The model under review builds one solid part; all positions refer to its coordinate system, in mm. Face numbers are marked on the shaded views. A direction names the side the tool comes from. Coordinates: 2 decimals unless noted, no trailing zeros. Order: outer loops, then holes, each group sorted by start corner. A loop starts at its lowest first (then second) coordinate and runs counter-clockwise, first axis right, second up. Notation, with made-up numbers: (-26, -15) -> (-17, -15) arc R12 ccw to (-17, 0) -> close; hole circle Ø7 at (51, -39.5). An arc over 180 degrees is marked (long way). Use one line per item in the form item = value. Start each with the question number.
(1) Insertion check: pin 1 Ø10 at (x, z) = (14.5, -59) entering from -Y; pin 2 Ø2 at (x, y) = (-59.5, 17.5) entering from +Z (3 decimals); pin 3 Ø1.5 at (y, z) = (20.5, -4) entering from -X; pin 4 Ø0.5 at (x, y) = (59.5, 17.5) entering from -Z (3 decimals). Each pin has a flat end and moves straight along its axis. Give the tip position at first contact, or say it passes through.
(2) Take a section at D-D (z = 63). State the section outline as (x, y) points.
(3) Wall thickness on line 1 along X through (y, z) = (12.5, -47.5) (3 decimals); line 2 along X through (y, z) = (17, -27) (3 decimals); line 3 along Y through (x, z) = (47, 28): over which ranges is each line inside the solid? List them lowest first.
(4) Mouldability with a two-part tool opening along Z and no side actions: class the marked faces 4, 5 and 6 as +Z half, -Z half, draft (parallel to the pull), parting line (faces both ways), or undercut.
(5) Take a section at B-B (x = 7.5). State the section outline as (y, z) points (3 decimals), then the cut area to 3 significant figures.
(6) Take a section at A-A (z = 24). State the section outline as (x, y) points (3 decimals).
(7) Take a section at C-C (x = 47). State the section outline as (y, z) points (3 decimals), then the cut area to 3 significant figures.
(8) For the marked faces 1, 2 and 3, list the 3-axis set-ups (+Z, -Z, +X, -X, +Y, -Y) from which the entire face can be reached by the end or side of a thin tool; tool diameter is ignored.
```python
from build123d import *

# Parameters (mm, degrees)
BOSS_EXTRUDE1_DEPTH     = 6.35
SKETCH3_W               = 120.65
SKETCH3_H               = 120.65
SKETCH3_W_2             = 107.95
SKETCH3_H_2             = 114.3
BOSS_EXTRUDE2_DEPTH     = 19.558
FILLET2_R               = 3.81
CUT_EXTRUDE2_DEPTH      = 52.07
CUT_EXTRUDE2_DEPTH_BACK = 39.37
FILLET3_R               = 3.81
CHAMFER1_SIZE           = 2.54


with BuildPart() as part:
    # Sketch2 → Boss-Extrude1 (new body)
    with BuildSketch(Plane(origin=(0, 0, 0), x_dir=(1, 0, 0), z_dir=(0, 1, 0))):
        with BuildLine():
            ThreePointArc((-76.2, 34.925), (-73.750256121, 26.470795103), (-66.04, 22.225))
            ThreePointArc((-66.04, 22.225), (-71.103893825, 18.75335434), (-73.66, 13.171090867))
            Line((-73.66, 13.171090867), (-73.66, -53.975))
            ThreePointArc((-73.66, -53.975), (-68.080384182, -67.445384182), (-54.61, -73.025))
            Line((-54.61, -73.025), (54.61, -73.025))
            ThreePointArc((54.61, -73.025), (68.080384182, -67.445384182), (73.66, -53.975))
            Line((73.66, -53.975), (73.66, 9.525))
            ThreePointArc((73.66, 9.525), (72.166535166, 17.2649211), (66.04, 22.225))
            ThreePointArc((66.04, 22.225), (73.750256121, 26.470795103), (76.2, 34.925))
            add(Edge.make_bspline(
                [(54.26154132, 73.334062346), (78.033661383, 68.772092229), (76.2, 34.925)],
                knots=[0, 0, 0, 1, 1, 1], degree=2))
            ThreePointArc((54.26154132, 73.334062346), (0, 79.119757765), (-54.26154132, 73.334062346))
            add(Edge.make_bspline(
                [(-54.26154132, 73.334062346), (-78.033661383, 68.772092229), (-76.2, 34.925)],
                knots=[0, 0, 0, 1, 1, 1], degree=2))
        make_face()
    extrude(amount=BOSS_EXTRUDE1_DEPTH)

    # Sketch3 → Boss-Extrude2 (add)
    with BuildSketch(Plane(origin=(0, 6.35, 0), x_dir=(1, 0, 0), z_dir=(0, 1, 0))):
        Rectangle(SKETCH3_W, SKETCH3_H)
        Rectangle(SKETCH3_W_2, SKETCH3_H_2, mode=Mode.SUBTRACT)
    extrude(amount=BOSS_EXTRUDE2_DEPTH)

    # Fillet2
    fillet2_edges = [part.edges().sort_by_distance(p)[0] for p in [
        (53.975, 6.35, 0),
        (0, 6.35, -57.15),
        (-53.975, 6.35, 0),
        (0, 6.35, 57.15),
    ]]
    fillet(fillet2_edges, radius=FILLET2_R)

    # Sketch5 → Cut-Extrude2 (cut, two sides: drawn at the far end of the back side and taken through both)
    with BuildSketch(Plane.XY.offset(-CUT_EXTRUDE2_DEPTH_BACK)):
        with BuildLine():
            Line((60.325, 21.4247353), (60.325, 12.6112647))
            ThreePointArc((60.325, 12.6112647), (58.547, 17.018), (60.325, 21.4247353))
        make_face()
        with BuildLine():
            Line((-60.325, 21.4247353), (-60.325, 12.6112647))
            ThreePointArc((-60.325, 12.6112647), (-58.547, 17.018), (-60.325, 21.4247353))
        make_face()
    extrude(amount=CUT_EXTRUDE2_DEPTH + CUT_EXTRUDE2_DEPTH_BACK, mode=Mode.SUBTRACT)

    # Fillet3
    # the kernel refuses this fillet: 3.81 mm, written as the material it adds along each edge
    with BuildSketch(Plane(origin=(-50.165, 10.16, 53.34), x_dir=(0, 0, 1), z_dir=(-1, 0, 0))) as fillet3_piece_1_section:
        Polygon((0, 0), (FILLET3_R, 0), (FILLET3_R, -FILLET3_R), (0, -FILLET3_R), align=None)
    fillet3_piece_1 = extrude(amount=FILLET3_R, mode=Mode.PRIVATE)
    fillet3_piece_1 = fillet3_piece_1 - Plane(origin=(-50.165, 10.16, 53.34), x_dir=(0, 0.7071067811865475, -0.7071067811865475), z_dir=(-1, 0, 0)) * Sphere(FILLET3_R, mode=Mode.PRIVATE)
    add(fillet3_piece_1)
    with BuildSketch(Plane(origin=(-50.165, 10.16, -53.34), x_dir=(0, 0, -1), z_dir=(-1, 0, 0))) as fillet3_piece_2_section:
        Polygon((0, 0), (FILLET3_R, 0), (FILLET3_R, FILLET3_R), (0, FILLET3_R), align=None)
    fillet3_piece_2 = extrude(amount=FILLET3_R, mode=Mode.PRIVATE)
    fillet3_piece_2 = fillet3_piece_2 - Plane(origin=(-50.165, 10.16, -53.34), x_dir=(0, 0.7071067811865475, 0.7071067811865475), z_dir=(-1, 0, 0)) * Sphere(FILLET3_R, mode=Mode.PRIVATE)
    add(fillet3_piece_2)
    with BuildSketch(Plane(origin=(50.165, 10.16, 53.34), x_dir=(1, 0, 0), z_dir=(0, 0, 1))) as fillet3_piece_3_section:
        Polygon((0, 0), (FILLET3_R, 0), (FILLET3_R, -FILLET3_R), (0, -FILLET3_R), align=None)
    fillet3_piece_3 = extrude(amount=FILLET3_R, mode=Mode.PRIVATE)
    fillet3_piece_3 = fillet3_piece_3 - Plane(origin=(50.165, 10.16, 53.34), x_dir=(-0.7071067811865475, 0.7071067811865475, 0), z_dir=(0, 0, 1)) * Sphere(FILLET3_R, mode=Mode.PRIVATE)
    add(fillet3_piece_3)
    with BuildSketch(Plane(origin=(50.165, 10.16, -53.34), x_dir=(1, 0, 0), z_dir=(0, 0, -1))) as fillet3_piece_4_section:
        Polygon((0, 0), (FILLET3_R, 0), (FILLET3_R, FILLET3_R), (0, FILLET3_R), align=None)
    fillet3_piece_4 = extrude(amount=FILLET3_R, mode=Mode.PRIVATE)
    fillet3_piece_4 = fillet3_piece_4 - Plane(origin=(50.165, 10.16, -53.34), x_dir=(-0.7071067811865475, 0.7071067811865475, 0), z_dir=(0, 0, -1)) * Sphere(FILLET3_R, mode=Mode.PRIVATE)
    add(fillet3_piece_4)
    with BuildSketch(Plane(origin=(53.975, 10.16, -57.15), x_dir=(-1, 0, 0), z_dir=(0, 1, 0)), Plane(origin=(-53.975, 10.16, -57.15), x_dir=(0, 0, 1), z_dir=(0, 1, 0))) as fillet3_piece_5:
        with BuildLine():
            CenterArc((FILLET3_R, FILLET3_R), FILLET3_R, 180, 90)
            Line((0, FILLET3_R), (0, 0))
            Line((0, 0), (FILLET3_R, 0))
        make_face()
    extrude(amount=15.748)
    with BuildSketch(Plane(origin=(-53.975, 10.16, 57.15), x_dir=(0, 0, -1), z_dir=(0, 1, 0)), Plane(origin=(53.975, 10.16, 57.15), x_dir=(-1, 0, 0), z_dir=(0, 1, 0))) as fillet3_piece_6:
        with BuildLine():
            CenterArc((FILLET3_R, -FILLET3_R), FILLET3_R, 90, 90)
            Line((0, -FILLET3_R), (0, 0))
            Line((0, 0), (FILLET3_R, 0))
        make_face()
    extrude(amount=15.748)

    # Chamfer1
    chamfer1_edges = [part.edges().sort_by_distance(p)[0] for p in [
        (60.325, 25.908, 0),
        (0, 25.908, -60.325),
        (-60.325, 25.908, 0),
        (0, 25.908, 60.325),
    ]]
    chamfer(chamfer1_edges, length=CHAMFER1_SIZE)


solid = part.part
```
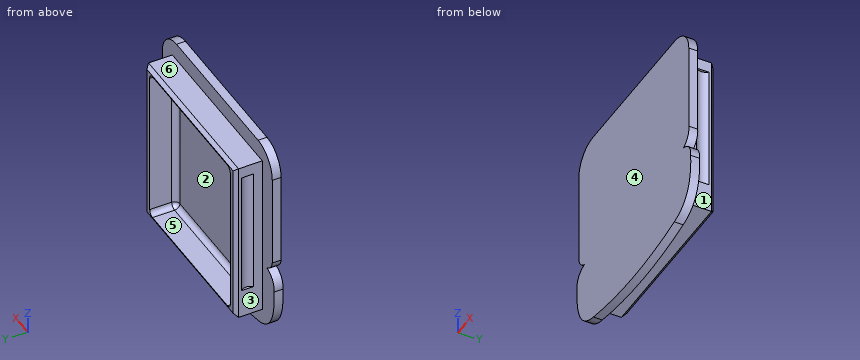
Findings:
q1.pin_1 = 0
q1.pin_2 = 60.325
q1.pin_3 = -60.16
q1.pin_4 = -60.325
q2.outline = (-71.39, 0) -> (71.39, 0) -> (71.39, 6.35) -> (-71.39, 6.35) -> close
q3.line_1 = -60.325 to -53.975, 53.975 to 60.325
q3.line_2 = -58.547 to -53.975, 53.975 to 58.547
q3.line_3 = 0 to 6.35
q4.face_4 = draft
q4.face_5 = undercut
q4.face_6 = +Z half
q5.outline = (0, -79.01) -> (6.35, -79.01) -> (6.35, -60.325) -> (23.368, -60.325) -> (25.908, -57.785) -> (25.908, -57.15) -> (10.16, -57.15) arc R3.81 cw to (6.35, -53.34) -> (6.35, 53.34) arc R3.81 cw to (10.16, 57.15) -> (25.908, 57.15) -> (25.908, 57.785) -> (23.368, 60.325) -> (6.35, 60.325) -> (6.35, 73.025) -> (0, 73.025) -> close
q5.area = 1,090 mm²
q6.outline = (-73.66, 0) -> (73.66, 0) -> (73.66, 6.35) -> (60.325, 6.35) -> (60.325, 12.611) arc R6.35 cw to (60.325, 21.425) -> (60.325, 23.368) -> (57.785, 25.908) -> (53.975, 25.908) -> (53.975, 10.16) arc R3.81 cw to (50.165, 6.35) -> (-50.165, 6.35) arc R3.81 cw to (-53.975, 10.16) -> (-53.975, 25.908) -> (-57.785, 25.908) -> (-60.325, 23.368) -> (-60.325, 21.425) arc R6.35 cw to (-60.325, 12.611) -> (-60.325, 6.35) -> (-73.66, 6.35) -> close
q7.outline = (0, -74.791) -> (6.35, -74.791) -> (6.35, -60.325) -> (23.368, -60.325) -> (25.908, -57.785) -> (25.908, -57.15) -> (10.16, -57.15) arc R3.81 cw to (6.35, -53.34) -> (6.35, 53.34) arc R3.81 cw to (10.16, 57.15) -> (25.908, 57.15) -> (25.908, 57.785) -> (23.368, 60.325) -> (6.35, 60.325) -> (6.35, 73.025) -> (0, 73.025) -> close
q7.area = 1,060 mm²
q8.face_1 = +Z, -Z, +X, +Y
q8.face_2 = +Y
q8.face_3 = +Z, -Z, -X, +Y
